Geometry: see drawing. Coordinates: mm, zero at the bounding-box minimum. A direction names the side the tool comes from. Coordinates: 2 decimals unless noted, no trailing zeros. Order: outer loops, then holes, each group sorted by start corner. A loop starts at its lowest first (then second) coordinate and runs counter-clockwise, first axis right, second up.
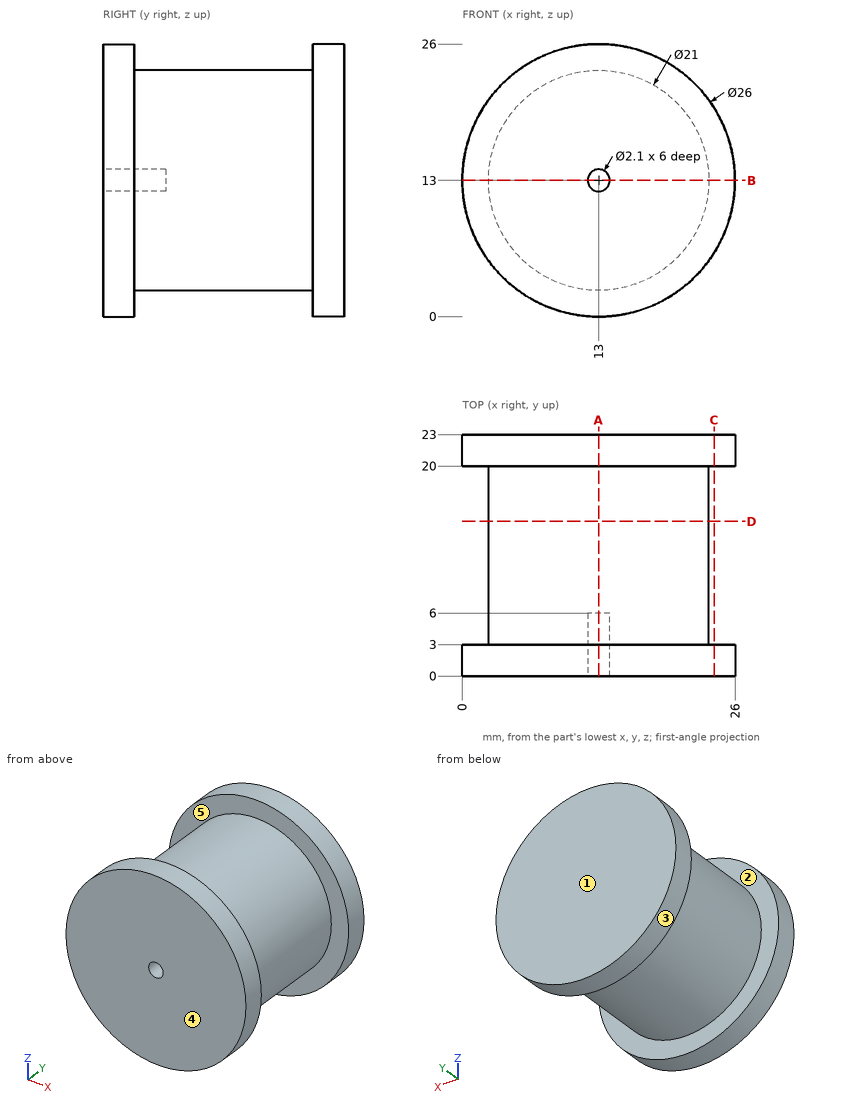
Q1. Section query C-C on x = 24. Output: boundary loops of the cut face in (y, z), plus the area to 3 significant figures.
Solutions:
outline: (0, 6.07) - (3, 6.07) - (3, 19.93) - (0, 19.93) - close; (20, 6.07) - (23, 6.07) - (23, 19.93) - (20, 19.93) - close
area: 83.1 mm2
Q2. Section query B-B on z = 13. Output: boundary loops of the cut face in (x, y).
Solutions:
outline: (0, 0) - (11.95, 0) - (11.95, 6) - (14.05, 6) - (14.05, 0) - (26, 0) - (26, 3) - (23.5, 3) - (23.5, 20) - (26, 20) - (26, 23) - (0, 23) - (0, 20) - (2.5, 20) - (2.5, 3) - (0, 3) - close
Q3. Material intervals for line 1 along Z through (x, y) = (13, 1.8); line 2 along Y through (x, z) = (22.5, 5.75); line 3 along Z through (x, y) = (13, 3.2), sorted ascending.
Solutions:
line 1: z = 0 to 11.95, 14.05 to 26
line 2: y = 0 to 3, 20 to 23
line 3: z = 2.5 to 11.95, 14.05 to 23.5
Q4. Set-up query: the marked faces 4 and 5. Return all of +Z, -Z, +X, -X, +Y, -Y with unobstructed straight access to the full face (end or side cutting, diameter ignored); none if empty.
Solutions:
face 4: +Z, -Z, +X, -X, -Y
face 5: none
Q5. Pull-direction query (Y, two-part tool) for the marked faces 1, 2 and 3; classes: pulls with the +Y half, pulls with the -Y half, needs draft (parallel to the pull), parting line crosses it, or undercut.
Solutions:
face 1: pulls with the +Y half
face 2: undercut
face 3: needs draft
Q6. Pin query (flat end, axial travel): P1, Ø3, axis at y = 12, z = 11, coming from the -X side; P2, Ø1.5, axis at y = 16, z = 16, coming from the -X side; P3, Ø2, axis at x = 11.5, y = 12, coming from the +Z side. Return the tip coordinate at first contact, or that it passes through.
Solutions:
P1: stops at x = 2.51
P2: stops at x = 2.74
P3: stops at z = 23.49
Q7. Section query D-D on y = 14.75. Output: boundary loops of the cut face in (x, z).
Solutions:
outline: circle Ø21 at (13, 13)
Q8. Section query A-A on x = 13. Output: boundary loops of the cut face in (y, z).
Solutions:
outline: (0, 0) - (3, 0) - (3, 2.5) - (20, 2.5) - (20, 0) - (23, 0) - (23, 26) - (20, 26) - (20, 23.5) - (3, 23.5) - (3, 26) - (0, 26) - (0, 14.05) - (6, 14.05) - (6, 11.95) - (0, 11.95) - close
